The model under review builds one solid part; all positions refer to its coordinate system, in mm. A direction names the side the tool comes from. Give positions to 0.01 mm unless a question says otherwise; leave off trailing zeros. Loops run counter-clockwise (first coordinate to the right, second up) from the corner with the lowest first, then second, coordinate; pieces in that order, holes last. Notation, with made-up numbers: M 0.5,-2.5 L 28.5,-2.5 A11 cw 28.5,1.5 Z; hole C 71,35.25 d3. An arc over 180 degrees is marked long. Return JSON: item names as keys, results as strings.
```python
from build123d import *

# Parameters (mm, degrees)
SKETCH_2_W             = 28
SKETCH_2_H             = 4.5
CUT_EXTRUDE_1_DEPTH    = 10
EXTRUDE_1_DEPTH        = 15
HOLE_WIZARD_M3_1_D     = 2.5
HOLE_WIZARD_M3_1_DEPTH = 4
HOLE_WIZARD_M3_1_TIP   = 0.751075774
CUT_EXTRUDE_START      = -20
CUT_EXTRUDE_2_DEPTH    = 20
HOLE_WIZARD_M4_1_D     = 3.3
HOLE_WIZARD_M4_1_DEPTH = 10.1
HOLE_WIZARD_M4_1_TIP   = 0.991420021


with BuildPart() as part:
    # 草图1 → 旋转1 (revolve)
    with BuildSketch(Plane.XY, mode=Mode.PRIVATE) as revolve_1_sk:
        Polygon((0, 0), (4.1, 0), (4.1, 6.7), (13.4, 6.7), (13.4, 8.7), (21, 8.7), (21, 10.2), (20, 10.2), (20, 11.2), (21, 11.2), (21, 12.2), (10, 12.2), (10, 13.2), (21, 13.2), (21, 20.4), (5, 20.4), (5, 21), (21, 21), (21, 34.7), (18.3, 38.7), (3.5, 38.7), (3.5, 43.7), (0, 43.7), align=None)
    revolve(revolve_1_sk.sketch.rotate(Axis((0, 43.7, 0), (0, -1, 0)), 90), axis=Axis((0, 43.7, 0), (0, -1, 0)))

    # 草图2 → 切除-拉伸1 (cut)
    with BuildSketch(Plane.XY.offset(21)):
        with Locations((0, 16.05)):
            Rectangle(SKETCH_2_W, SKETCH_2_H)
    extrude(amount=-CUT_EXTRUDE_1_DEPTH, mode=Mode.SUBTRACT)

    # 草图3 → 凸台-拉伸1 (add)
    with BuildSketch(Plane.XY.offset(11)):
        with BuildLine():
            Line((9.185056323, 18.053194417), (9.385056323, 18.053194417))
            ThreePointArc((9.385056323, 18.053194417), (11.385056323, 16.053194417), (9.385056323, 14.053194417))
            Line((9.385056323, 14.053194417), (9.185056323, 14.053194417))
            ThreePointArc((9.185056323, 14.053194417), (7.185056323, 16.053194417), (9.185056323, 18.053194417))
        make_face()
    extrude(amount=EXTRUDE_1_DEPTH)

    # M3 螺纹孔1
    with Locations(Plane(origin=(0, 38.7, 0), x_dir=(1, 0, 0), z_dir=(0, 1, 0))):
        with Locations((-6.5, 0), (6.5, 0)):
            Hole(HOLE_WIZARD_M3_1_D / 2, depth=HOLE_WIZARD_M3_1_DEPTH)
            with Locations((0, 0, -(HOLE_WIZARD_M3_1_DEPTH + HOLE_WIZARD_M3_1_TIP / 2))):  # 118° drill point
                Cone(0, HOLE_WIZARD_M3_1_D / 2, HOLE_WIZARD_M3_1_TIP, mode=Mode.SUBTRACT)

    # 草图7 → 旋转2 (revolve)
    with BuildSketch(Plane.XY, mode=Mode.PRIVATE) as revolve_2_sk:
        Polygon((0, -55.3), (5, -55.3), (5, -31.2), (8.275, -31.2), (8.275, -30.3), (13, -30.3), (13, -28.3), (21, -28.3), (21, 8.7), (0, 8.7), align=None)
    revolve(revolve_2_sk.sketch.rotate(Axis((0, 8.7, 0), (0, -1, 0)), 180), axis=Axis((0, 8.7, 0), (0, -1, 0)))

    # 草图8 → 切除-拉伸2 (cut)
    with BuildSketch(Plane.XZ.offset(55.3).offset(CUT_EXTRUDE_START)):
        with BuildLine():
            Line((-3, 4), (3, 4))
            ThreePointArc((3, 4), (0, 5), (-3, 4))
        make_face()
    extrude(amount=CUT_EXTRUDE_2_DEPTH, mode=Mode.SUBTRACT)

    # M4 螺纹孔1
    with Locations(Plane(origin=(0, -28.3, 0), x_dir=(-1, 0, 0), z_dir=(0, -1, 0))):
        with Locations((17.5, 0), (0, -17.5), (-17.5, 0), (0, 17.5)):
            Hole(HOLE_WIZARD_M4_1_D / 2, depth=HOLE_WIZARD_M4_1_DEPTH)
            with Locations((0, 0, -(HOLE_WIZARD_M4_1_DEPTH + HOLE_WIZARD_M4_1_TIP / 2))):  # 118° drill point
                Cone(0, HOLE_WIZARD_M4_1_D / 2, HOLE_WIZARD_M4_1_TIP, mode=Mode.SUBTRACT)


solid = part.part
```
1) Consider section A-A on y = -26. Write out the cut boundary in (x, z), then the cut area to 3 significant figures.
From the geometry:
{"outline": "C 0,0 d42; hole C -17.5,0 d3.3; hole C 0,-17.5 d3.3; hole C 0,17.5 d3.3; hole C 17.5,0 d3.3", "area": "1,350 mm²"}
2) The part is to be moulded in two halves that separate along Z. For faces 6 (the face through (8, 11.2, -19)), 7 (the face through (-5.25, 36.67, -0.05)), 8 (the face through (3.105, 41.235, 1.615)), say which applies: released by +Z, released by -Z, zero draft, split by the parting line, or undercut.
From the geometry:
{"face 6": "zero draft", "face 7": "undercut", "face 8": "split by the parting line"}
3) Insertion check: pin 1 (10 mm diameter, centred on x = 14.5, y = 10.5, fed in from -Z); pin 2 (5 mm diameter, centred on y = -16.5, z = 8, fed in from +X); pin 3 (8 mm diameter, centred on x = 6.5, z = 15.5, fed in from -Y); pin 4 (12.5 mm diameter, centred on x = -6, z = 1, fed in from -Y). Each pin has a flat end and moves straight along its axis. Give the tip position at first contact, or say it passes through.
From the geometry:
{"pin 1": "z = -18.72", "pin 2": "x = 20.27", "pin 3": "y = -30.3", "pin 4": "y = -55.3"}
4) Tool access review of faces 1 (the face through (0, 43.7, 0)), 2 (the face through (-0.2, -30.3, 8.5)), 3 (the face through (14, 16, 13)), 4 (the face through (9, 16, 26)), 5 (the face through (4, 21, -4)): name each direction out of +Z, -Z, +X, -X, +Y, -Y from which nothing blocks a thin tool from reaching the whole face with its end or side.
From the geometry:
{"face 1": "+Z, -Z, +X, -X, +Y", "face 2": "-Y", "face 3": "+Z", "face 4": "+Z, +X, -X, +Y, -Y", "face 5": "none"}
5) Wall thickness on L1, parallel to Y at x = -14, z = 2.5; L2, parallel to Y at x = -7, z = 10.5; L3, parallel to Y at x = -5.5, z = 4: over which ranges is each line inside the solid? List them lowest first. Write a range as from..to.
From the geometry:
{"L1": "-28.3..12.2, 13.2..20.4, 21..38.7", "L2": "-30.3..12.2, 13.2..20.4, 21..38.7", "L3": "-31.2..20.4, 21..38.7"}
6) Consider section B-B on y = -44. Write out the cut boundary in (x, z).
From the geometry:
{"outline": "M -3,4 A5 ccw long 3,4 Z"}
7) Consider section C-C on y = -9.5. Write out the cut boundary in (x, z).
From the geometry:
{"outline": "C 0,0 d42"}
